Check sheet for the drawn part. Datum: minimum x, y, z corner. Units: mm. Round coordinates to 2 decimals unless told otherwise and drop trailing zeros. Write each loop counter-clockwise with the first axis right and the second up, starting at its lowest first coordinate (ties: lowest second). Pieces come first, ordered by that corner, then holes. Notation, with made-up numbers: M -9,65 L 15,65 A18 cw 15,84 Z; hole C 85.5,70 d11. An arc over 180 degrees is marked long. Use a Markdown table: item, result.
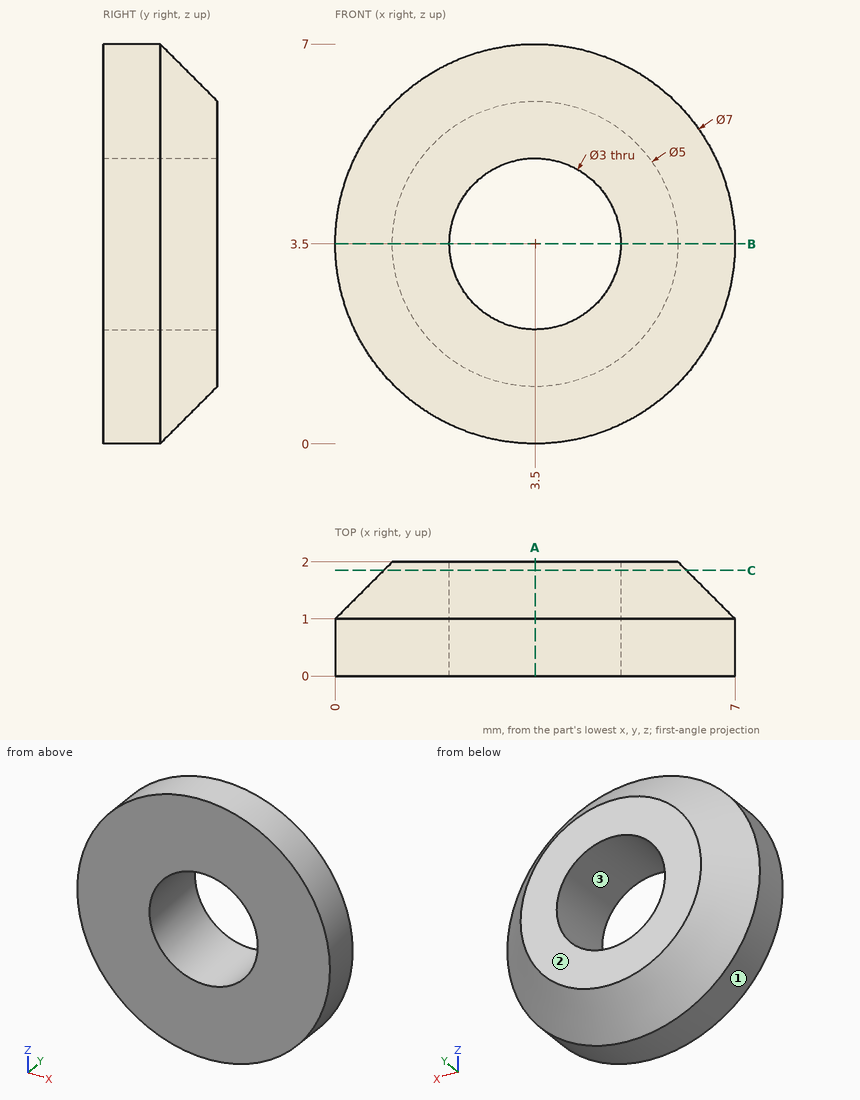
Item 1: Cross-section at A-A, the plane x = 3.5. Record the cut outline in (y, z).
Outcome:
| item | result |
|---|---|
| outline | M 0,0 L 1,0 L 2,1 L 2,2 L 0,2 Z; M 0,5 L 2,5 L 2,6 L 1,7 L 0,7 Z |
Item 2: Mould release check, pull along Z, two halves, no side actions. Record for the marked faces 1, 2 and 3: +Z half, -Z half, draft (parallel to the pull), parting line (faces both ways), or undercut.
Outcome:
| item | result |
|---|---|
| face 1 | parting line |
| face 2 | draft |
| face 3 | undercut |
Item 3: Go/stop test with a flat-tipped pin: pin 1 (2 mm diameter, centred on x = 4.5, z = 1.5, fed in from -Y). Record where the tip stops, or that it passes through.
Outcome:
| item | result |
|---|---|
| pin 1 | stops at y = 0 |
Item 4: Cross-section at C-C, the plane y = 1.85. Record the cut outline in (x, z).
Outcome:
| item | result |
|---|---|
| outline | C 3.5,3.5 d5.3; hole C 3.5,3.5 d3 |
Item 5: Cross-section at B-B, the plane z = 3.5. Record the cut outline in (x, y).
Outcome:
| item | result |
|---|---|
| outline | M 0,0 L 2,0 L 2,2 L 1,2 L 0,1 Z; M 5,0 L 7,0 L 7,1 L 6,2 L 5,2 Z |
Item 6: Material ranges on line 1 along Z through (x, y) = (3.5, 0.95); line 2 along Z through (x, y) = (3.5, 1.6), recorded low to high. Write a range as from..to.
Outcome:
| item | result |
|---|---|
| line 1 | z = 0..2, 5..7 |
| line 2 | z = 0.6..2, 5..6.4 |
